```python
from build123d import *

# Parameters (mm, degrees)
SKETCH1_W           = 150
SKETCH1_H           = 150
SKETCH1_W_2         = 15
SKETCH1_H_2         = 75
BOSS_EXTRUDE1_DEPTH = 5
SKETCH2_R           = 1.5
SKETCH2_R_2         = 10
SKETCH2_W           = 14
SKETCH2_H           = 3
CUT_EXTRUDE1_DEPTH  = 5


with BuildPart() as part:
    # Sketch1 → Boss-Extrude1 (new body)
    with BuildSketch(Plane(origin=(0, 0, 0), x_dir=(1, 0, 0), z_dir=(0, 1, 0))):
        Rectangle(SKETCH1_W, SKETCH1_H)
        with Locations((-50, 0)):
            Rectangle(SKETCH1_W_2, SKETCH1_H_2, mode=Mode.SUBTRACT)
        with Locations((50, 0)):
            Rectangle(SKETCH1_W_2, SKETCH1_H_2, mode=Mode.SUBTRACT)
    extrude(amount=BOSS_EXTRUDE1_DEPTH)

    # Sketch2 → Cut-Extrude1 (cut)
    with BuildSketch(Plane(origin=(0, 5, 0), x_dir=(1, 0, 0), z_dir=(0, 1, 0))):
        with Locations((-50, 60)):
            Circle(SKETCH2_R)
        with Locations((50, 60)):
            Circle(SKETCH2_R)
        with Locations((0, 45)):
            Circle(SKETCH2_R_2)
        Circle(SKETCH2_R)
        with Locations((-17.5, 25.75)):
            Rectangle(SKETCH2_W, SKETCH2_H)
        with Locations((17.5, 25.75)):
            Rectangle(SKETCH2_W, SKETCH2_H)
        with Locations((-17.5, -25.75)):
            Rectangle(SKETCH2_W, SKETCH2_H)
        with Locations((17.5, -25.75)):
            Rectangle(SKETCH2_W, SKETCH2_H)
    extrude(amount=-CUT_EXTRUDE1_DEPTH, mode=Mode.SUBTRACT)


solid = part.part
```
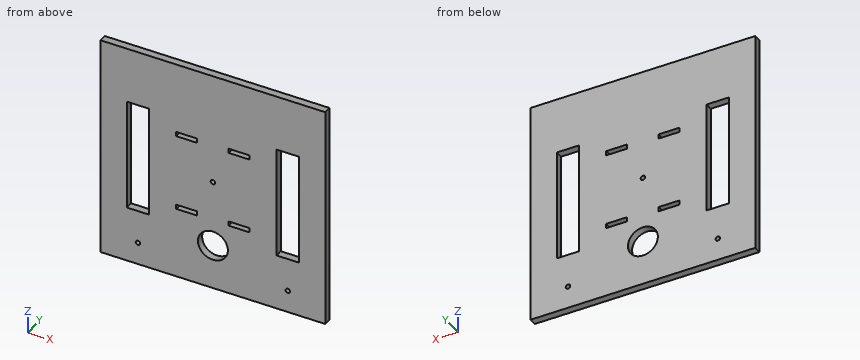
CAD build for the part. Positions are in the model's coordinates, mm. Round coordinates to 2 decimals unless told otherwise and drop trailing zeros. Order: outer loops, then holes, each group sorted by start corner. A loop starts at its lowest first (then second) coordinate and runs counter-clockwise, first axis right, second up.
Item 1: Saw through at C-C on z = -45. Write the cut outline in (x, y), then the cut area to 3 significant figures.
Item 2: Saw through at B-B on x = 55. Write the cut outline in (y, z).
Item 3: Pin check, flat tip, straight feed: pin 1 (2.5 mm diameter, centred on x = 50, z = -60, fed in from -Y) (3 decimals). Stop position of the tip, or through.
Item 4: Saw through at D-D on x = 16.5. Write the cut outline in (y, z).
Item 5: Saw through at A-A on z = 10.5. Write the cut outline in (x, y), then the cut area to 3 significant figures.
Item 6: Probe line 1 along X through (y, z) = (3.65, -32.5); line 2 along Z through (x, y) = (50, 1.75); line 3 along Z through (x, y) = (0, 1.5). List the from-to ranges inside material, lowest first.
Reported:
1. outline: (-75, 0) - (-10, 0) - (-10, 5) - (-75, 5) - close; (10, 0) - (75, 0) - (75, 5) - (10, 5) - close
1. area: 650 mm2
2. outline: (0, -75) - (5, -75) - (5, -37.5) - (0, -37.5) - close; (0, 37.5) - (5, 37.5) - (5, 75) - (0, 75) - close
3. pin 1: passes through
4. outline: (0, -75) - (5, -75) - (5, -27.25) - (0, -27.25) - close; (0, -24.25) - (5, -24.25) - (5, 24.25) - (0, 24.25) - close; (0, 27.25) - (5, 27.25) - (5, 75) - (0, 75) - close
5. outline: (-75, 0) - (-57.5, 0) - (-57.5, 5) - (-75, 5) - close; (-42.5, 0) - (42.5, 0) - (42.5, 5) - (-42.5, 5) - close; (57.5, 0) - (75, 0) - (75, 5) - (57.5, 5) - close
5. area: 600 mm2
6. line 1: x = -75 to -57.5, -42.5 to 42.5, 57.5 to 75
6. line 2: z = -75 to -61.5, -58.5 to -37.5, 37.5 to 75
6. line 3: z = -75 to -55, -35 to -1.5, 1.5 to 75
